from build123d import *

# Parameters (mm, degrees)
CROQUIS1_R              = 2.75
CROQUIS1_R_2            = 0.2
SALIENTE_EXTRUIR1_DEPTH = 0.25
SALIENTE_EXTRUIR2_DEPTH = 0.25
MATRIZC1_COUNT          = 15


with BuildPart() as part:
    # Croquis1 → Saliente-Extruir1 (new body)
    with BuildSketch(Plane.XY):
        Circle(CROQUIS1_R)
        Circle(CROQUIS1_R_2, mode=Mode.SUBTRACT)
        with BuildLine():
            Line((0.125, -2.496873044), (0.125, -0.739509973))
            ThreePointArc((0.125, -0.739509973), (0.530330086, -0.530330086), (0.739509973, -0.125))
            Line((0.739509973, -0.125), (2.496873044, -0.125))
            ThreePointArc((2.496873044, -0.125), (1.767766953, -1.767766953), (0.125, -2.496873044))
        make_face(mode=Mode.SUBTRACT)
        with BuildLine():
            ThreePointArc((-0.125, 2.496873044), (-1.767766953, 1.767766953), (-2.496873044, 0.125))
            Line((-2.496873044, 0.125), (-0.739509973, 0.125))
            ThreePointArc((-0.739509973, 0.125), (-0.530330086, 0.530330086), (-0.125, 0.739509973))
            Line((-0.125, 0.739509973), (-0.125, 2.496873044))
        make_face(mode=Mode.SUBTRACT)
        with BuildLine():
            Line((0.739509973, 0.125), (2.496873044, 0.125))
            ThreePointArc((2.496873044, 0.125), (1.767766953, 1.767766953), (0.125, 2.496873044))
            Line((0.125, 2.496873044), (0.125, 0.739509973))
            ThreePointArc((0.125, 0.739509973), (0.530330086, 0.530330086), (0.739509973, 0.125))
        make_face(mode=Mode.SUBTRACT)
        with BuildLine():
            Line((-2.496873044, -0.125), (-0.739509973, -0.125))
            ThreePointArc((-0.739509973, -0.125), (-0.530330086, -0.530330086), (-0.125, -0.739509973))
            Line((-0.125, -0.739509973), (-0.125, -2.496873044))
            ThreePointArc((-0.125, -2.496873044), (-1.767766953, -1.767766953), (-2.496873044, -0.125))
        make_face(mode=Mode.SUBTRACT)
    extrude(amount=SALIENTE_EXTRUIR1_DEPTH)

    # Croquis2 → Saliente-Extruir2 (add)
    with BuildSketch(Plane(origin=(0, 0, 0), x_dir=(-1, 0, 0), z_dir=(0, 0, -1))):
        with BuildLine():
            Line((-0.625, -3.613183026), (-0.4375, -3.721436201))
            Line((-0.4375, -3.721436201), (-0.477123412, -3.573559614))
            ThreePointArc((-0.477123412, -3.573559614), (-0.053677893, -2.999971472), (0.586755021, -2.686674254))
            ThreePointArc((0.586755021, -2.686674254), (0.232849703, -2.74012427), (-0.125, -2.747157622))
            Line((-0.125, -2.747157622), (-0.625, -3.613183026))
        make_face()
    saliente_extruir2 = extrude(amount=-SALIENTE_EXTRUIR2_DEPTH)

    # MatrizC1: Saliente-Extruir2 ×15 about axis
    matrizc1_axis = Axis((0, 0, 0), (0, 0, 1))
    for i in range(1, MATRIZC1_COUNT):
        add(saliente_extruir2.rotate(matrizc1_axis, i * 360 / MATRIZC1_COUNT))


solid = part.part
Geometry: final body of the model. Coordinates: model frame, mm. Give positions to 0.01 mm unless a question says otherwise; leave off trailing zeros. Order: outer loops, then holes, each group sorted by start corner. A loop starts at its lowest first (then second) coordinate and runs counter-clockwise, first axis right, second up. Notation, with made-up numbers: (43, 33) -> (89, 33) arc R19 ccw to (89, 69) -> close; hole circle Ø8 at (82.5, 37.25). An arc over 180 degrees is marked (long way). Answer as a JSON object with one key per item and string values.
Q1. Material intervals for probe 1 along Y at (x, z) = (-1.5, 0.1) (1 decimal); probe 2 along Y at (x, z) = (0, 0.2), sorted ascending.
Entries:
{"probe 1": "y = -2.3 to -2, -0.1 to 0.1, 2 to 2.4", "probe 2": "y = -2.96 to -0.2, 0.2 to 2.75"}
Q2. Section C-C (z = 0.2). State how many separate pieces and enclosed holes the cut face has, plus the area to 3 significant figures.
Entries:
{"separate pieces": "1", "enclosed holes": "5", "area": "10.2 mm^2"}
Q3. Section D-D (y = 0.5). Output: boundary loops of the cut face in (x, z).
Entries:
{"outline": "(-2.79, 0) -> (-2.45, 0) -> (-2.45, 0.25) -> (-2.79, 0.25) -> close; (-0.56, 0) -> (0.56, 0) -> (0.56, 0.25) -> (-0.56, 0.25) -> close; (2.45, 0) -> (2.7, 0) -> (2.7, 0.25) -> (2.45, 0.25) -> close; (2.84, 0) -> (3.08, 0) -> (3.08, 0.25) -> (2.84, 0.25) -> close"}
Q4. Section B-B (x = -0.5). Output: boundary loops of the cut face in (y, z), plus the area to 3 significant figures.
Entries:
{"outline": "(-2.71, 0) -> (-2.45, 0) -> (-2.45, 0.25) -> (-2.71, 0.25) -> close; (-0.56, 0) -> (0.56, 0) -> (0.56, 0.25) -> (-0.56, 0.25) -> close; (2.45, 0) -> (2.84, 0) -> (2.84, 0.25) -> (2.45, 0.25) -> close", "area": "0.443 mm^2"}
Q5. Section A-A (y = 2). Output: boundary loops of the cut face in (x, z) (3 decimals).
Entries:
{"outline": "(-1.887, 0) -> (-1.5, 0) -> (-1.5, 0.25) -> (-1.887, 0.25) -> close; (-0.125, 0) -> (0.125, 0) -> (0.125, 0.25) -> (-0.125, 0.25) -> close; (1.5, 0) -> (1.922, 0) -> (1.922, 0.25) -> (1.5, 0.25) -> close; (2.616, 0) -> (2.728, 0) -> (2.728, 0.25) -> (2.616, 0.25) -> close"}
